```python
from build123d import *

# Parameters (mm, degrees)
BOSS_EXTRUDE1_DEPTH = 15
CHAMFER1_SIZE       = 1
SKETCH2_R           = 1.75
CUT_EXTRUDE1_DEPTH  = 7


with BuildPart() as part:
    # Sketch1 → Boss-Extrude1 (new body)
    with BuildSketch(Plane.XY):
        Polygon((-9.662207358, 6), (17.337792642, 6), (17.337792642, -14.6), (10.337792642, -14.6), (10.337792642, 0), (-9.662207358, 0), align=None)
    extrude(amount=BOSS_EXTRUDE1_DEPTH)

    # Chamfer1
    chamfer1_edges = [part.edges().sort_by_distance(p)[0] for p in [
        (17.337792642, 6, 7.5),
    ]]
    chamfer(chamfer1_edges, length=CHAMFER1_SIZE)

    # Sketch2 → Cut-Extrude1 (cut, through all)
    with BuildSketch(Plane.XZ):
        with Locations((-4.662207358, 7.5)):
            Circle(SKETCH2_R)
        with Locations((5.337792642, 7.5)):
            Circle(SKETCH2_R)
    extrude(amount=-CUT_EXTRUDE1_DEPTH, mode=Mode.SUBTRACT)


solid = part.part
```
The listing builds one solid part. Answer for the finished solid, in the listing's coordinates (mm). A direction names the side the tool comes from. Coordinates: 2 decimals unless noted, no trailing zeros. Loops run counter-clockwise (first coordinate to the right, second up) from the corner with the lowest first, then second, coordinate; pieces in that order, holes last. Notation, with made-up numbers: M -10,-9.5 L -3,-9.5 A20 ccw -3,-3.5 Z; hole C -8,54 d5. An arc over 180 degrees is marked long. Answer as a JSON object with one key per item and string values. Group by question number.
Item 1: Section D-D (z = 13.25) is taken. Write down the section's boundary in (x, y), and give its area (3 significant figures).
Item 2: Section B-B (y = 2.5) is taken. Write down the section's boundary in (x, z), and give its area (3 significant figures).
Item 3: Section C-C (x = 6.5) is taken. Write down the section's boundary in (y, z), and give its area (3 significant figures).
Item 4: Section A-A (z = 7.5) is taken. Write down the section's boundary in (x, y).
Item 5: Which of the six approach directions +Z, -Z, +X, -X, +Y, -Y give full straight-line access (tool end or side, diameter ignored) to faces 4 (the face through (0, 0, 7)), 5 (the face through (-9.662, 3, 7))?
Item 6: Each of these flat-tipped pins is pushed along its axis until it touches: P1, Ø4.5, axis at x = 3, z = 8.5, coming from the -Y side; P2, Ø1, axis at y = -5.5, z = 6.5, coming from the -X side. Where does it stop, or does it pass through?
Item 7: Consider L1, parallel to X at y = 4.5, z = 6.5; L2, parallel to Y at x = 3.5, z = 7; L3, parallel to Z at x = -4.75, y = 2.5. Determine where each line is inside the solid, lowest interval first.
Item 8: Determine the mould class of faces 1 (the face through (14, -14.6, 7)), 2 (the face through (-6.41, 2.96, 7.58)), 3 (the face through (7, 0.4, 0)) for opening direction Z: +Z half, -Z half, draft (parallel to the pull), parting line (faces both ways), or undercut.
Solved:
{
 "1": {"outline": "M -9.66,0 L 10.34,0 L 10.34,-14.6 L 17.34,-14.6 L 17.34,5 L 16.34,6 L -9.66,6 Z", "area": "264 mm2"},
 "2": {"outline": "M -9.66,0 L 17.34,0 L 17.34,15 L -9.66,15 Z; hole C -4.66,7.5 d3.5; hole C 5.34,7.5 d3.5", "area": "386 mm2"},
 "3": {"outline": "M 0,0 L 6,0 L 6,6.19 L 0,6.19 Z; M 0,8.81 L 6,8.81 L 6,15 L 0,15 Z", "area": "74.3 mm2"},
 "4": {"outline": "M -9.66,0 L -6.41,0 L -6.41,6 L -9.66,6 Z; M -2.91,0 L 3.59,0 L 3.59,6 L -2.91,6 Z; M 7.09,0 L 10.34,0 L 10.34,-14.6 L 17.34,-14.6 L 17.34,5 L 16.34,6 L 7.09,6 Z"},
 "5": {"face 4": "+Z, -Z, -X, -Y", "face 5": "+Z, -Z, -X, +Y, -Y"},
 "6": {"P1": "stops at y = 0", "P2": "stops at x = 10.34"},
 "7": {"L1": "x = -9.66 to -6.1, -3.23 to 3.9, 6.77 to 17.34", "L2": "y = 0 to 6", "L3": "z = 0 to 5.75, 9.25 to 15"},
 "8": {"face 1": "draft", "face 2": "undercut", "face 3": "-Z half"}
}
